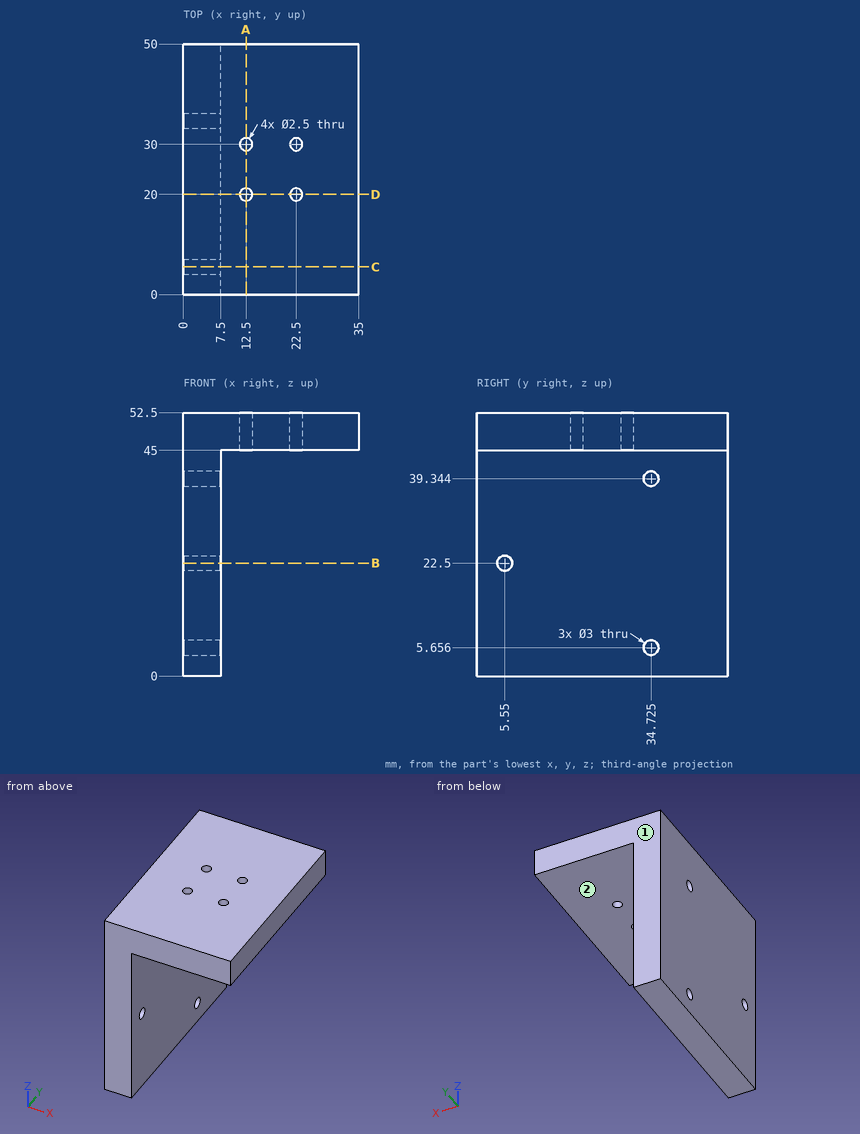
Source: three-view drawing plus pictorial views. Frame: mm from the lowest corner of the part. A direction names the side the tool comes from. Coordinates: 2 decimals unless noted, no trailing zeros. Loops run counter-clockwise (first coordinate to the right, second up) from the corner with the lowest first, then second, coordinate; pieces in that order, holes last. Notation, with made-up numbers: (22.5, 26) -> (30.5, 26) arc R33 cw to (30.5, 55) -> close; hole circle Ø5 at (68.5, 36.5). An arc over 180 degrees is marked (long way). Answer in a Markdown table with one row per item. Add a question column.
Q1. Section A-A on x = 12.5. Return the cut outline in (y, z).
Q2. Section D-D on y = 20. Return the cut outline in (x, z).
Q3. Ray query, line 1 along Y through (x, z) = (12.5, 50.25); line 2 along Y through (x, z) = (22, 47) (1 decimal); line 3 along Y through (x, z) = (3, 22.5). Return the intervals inside material, ascending.
Q4. Section C-C on y = 5.55. Return the cut outline in (x, z).
Q5. Contact query for flat-ended pins moving along their axis: pin 1 Ø5 at (y, z) = (26.5, 41) entering from +X; pin 2 Ø1.8 at (y, z) = (34.72, 5.66) entering from -X; pin 3 Ø3.5 at (y, z) = (34.72, 39.34) entering from -X; pin 4 Ø3 at (x, y) = (22.5, 20) entering from -Z. Output: stop coordinate, or through.
Q6. Reachability of the marked faces 1 and 2 from +Z, -Z, +X, -X, +Y, -Y: full face, straight path, thin tool, end or side. Return the list, or none.
Q7. Section B-B on z = 22.5. Return the cut outline in (x, y).
Computed values:
| question | item | result |
|---|---|---|
| 1 | outline | (0, 45) -> (18.75, 45) -> (18.75, 52.5) -> (0, 52.5) -> close; (21.25, 45) -> (28.75, 45) -> (28.75, 52.5) -> (21.25, 52.5) -> close; (31.25, 45) -> (50, 45) -> (50, 52.5) -> (31.25, 52.5) -> close |
| 2 | outline | (0, 0) -> (7.5, 0) -> (7.5, 45) -> (11.25, 45) -> (11.25, 52.5) -> (0, 52.5) -> close; (13.75, 45) -> (21.25, 45) -> (21.25, 52.5) -> (13.75, 52.5) -> close; (23.75, 45) -> (35, 45) -> (35, 52.5) -> (23.75, 52.5) -> close |
| 3 | line 1 | y = 0 to 18.75, 21.25 to 28.75, 31.25 to 50 |
| 3 | line 2 | y = 0 to 18.9, 21.1 to 28.9, 31.1 to 50 |
| 3 | line 3 | y = 0 to 4.05, 7.05 to 50 |
| 4 | outline | (0, 0) -> (7.5, 0) -> (7.5, 21) -> (0, 21) -> close; (0, 24) -> (7.5, 24) -> (7.5, 45) -> (35, 45) -> (35, 52.5) -> (0, 52.5) -> close |
| 5 | pin 1 | stops at x = 7.5 |
| 5 | pin 2 | passes through |
| 5 | pin 3 | stops at x = 0 |
| 5 | pin 4 | stops at z = 45 |
| 6 | face 1 | +Z, -Z, +X, -X, +Y |
| 6 | face 2 | -Z, +X, +Y, -Y |
| 7 | outline | (0, 0) -> (7.5, 0) -> (7.5, 4.05) -> (0, 4.05) -> close; (0, 7.05) -> (7.5, 7.05) -> (7.5, 50) -> (0, 50) -> close |
